For this review, take the finished solid that the model builds, in its own axes (mm). A direction names the side the tool comes from. Give positions to 0.01 mm unless a question says otherwise; leave off trailing zeros. Write each loop counter-clockwise with the first axis right and the second up, starting at its lowest first coordinate (ties: lowest second). Pieces come first, ordered by that corner, then holes. Notation, with made-up numbers: M -3.75,-36 L 35.25,-36 A33 cw 35.25,0 Z; hole C 72.5,80.25 d8. An arc over 180 degrees is marked long. Answer as a JSON object with one key per item and string values. Group by question number.
```python
from build123d import *

# Parameters (mm, degrees)
EXTRUDE_1_DEPTH     = 10
CUT_EXTRUDE_1_DEPTH = 3.6
SKETCH_3_R          = 4
CUT_EXTRUDE_2_DEPTH = 1.6


with BuildPart() as part:
    # Эскиз1 → Бобышка-Вытянуть1 (new body)
    with BuildSketch(Plane.XY):
        Polygon((2.5, 0), (-2.5, 0), (-5, 1.7), (-5, 3.7), (5, 3.7), (5, 1.7), align=None)
    extrude(amount=EXTRUDE_1_DEPTH)

    # Эскиз2 → Вырез-Вытянуть1 (cut)
    with BuildSketch(Plane(origin=(0, 3.7, 0), x_dir=(1, 0, 0), z_dir=(0, 1, 0))):
        Polygon((2.75, -6.58771324), (2.75, -3.41228676), (0, -1.824573519), (-2.75, -3.41228676), (-2.75, -6.58771324), (0, -8.175426481), align=None)
    extrude(amount=-CUT_EXTRUDE_1_DEPTH, mode=Mode.SUBTRACT)

    # Эскиз3 → Вырез-Вытянуть2 (cut)
    with BuildSketch(Plane(origin=(0, 3.7, 0), x_dir=(1, 0, 0), z_dir=(0, 1, 0))):
        with Locations(Location((0, -5, 0), (0, 0, 270))):
            Circle(SKETCH_3_R)
    extrude(amount=-CUT_EXTRUDE_2_DEPTH, mode=Mode.SUBTRACT)


solid = part.part
```
Item 1: Machinability: for faces 1 (the flat face through (-2.75, 1, 5)), 2 (the flat face through (-1, 2.1, 2)), 3 (the flat face through (-5, 3, 5)), which of the approach directions +Z, -Z, +X, -X, +Y, -Y give a long, thin tool a straight path to every point of the face, cutting with its end or side? Answer none if there is none.
Item 2: Consider section A-A (z = 5). Give the boundary of the cut face in (x, y).
Item 3: To check wall thickness, follow probe 1 along X at (y, z) = (3.25, 5); probe 2 along Y at (x, z) = (1.75, 2.5); probe 3 along X at (y, z) = (1.2, 5). State the ranges of each line that lie inside material, in increasing order.
Item 4: Consider section D-D (y = 1.2). Give the boundary of the cut face in (x, z).
Item 5: Draft analysis for pull direction X (two halves, no side actions). For faces 4 (the flat face through (0, 2, 10)), 5 (the flat face through (1.36, 1.11, 7.39)), 6 (the flat face through (5, 3, 5)), state which applies: released by +X, released by -X, zero draft, split by the parting line, or undercut.
Item 6: Consider section B-B (y = 1.95). Give the boundary of the cut face in (x, z), plus the area to 3 significant figures.
Item 7: Consider section C-C (x = 1). Give the boundary of the cut face in (y, z), plus the area to 3 significant figures.
Item 8: Insertion check: P1, Ø3, axis at x = 0, z = 5.5, coming from the +Y side. The pin has a flat end and moves straight along its axis. Give the tip position at first contact, or say it passes through.
Result set:
{
 "1": {"face 1": "+Y, -Y", "face 2": "+Y", "face 3": "+Z, -Z, -X, +Y, -Y"},
 "2": {"outline": "M -5,1.7 L -2.75,0.17 L -2.75,2.1 L -4,2.1 L -4,3.7 L -5,3.7 Z; M -2.65,0.1 L -2.5,0 L 2.5,0 L 2.65,0.1 Z; M 2.75,0.17 L 5,1.7 L 5,3.7 L 4,3.7 L 4,2.1 L 2.75,2.1 Z"},
 "3": {"probe 1": "x = -5 to -4, 4 to 5", "probe 2": "y = 0 to 2.1", "probe 3": "x = -4.26 to -2.75, 2.75 to 4.26"},
 "4": {"outline": "M -4.26,0 L 4.26,0 L 4.26,10 L -4.26,10 Z; hole M -2.75,3.41 L 0,1.82 L 2.75,3.41 L 2.75,6.59 L 0,8.18 L -2.75,6.59 Z"},
 "5": {"face 4": "zero draft", "face 5": "undercut", "face 6": "released by +X"},
 "6": {"outline": "M -5,0 L 5,0 L 5,10 L -5,10 Z; hole M -2.75,3.41 L 0,1.82 L 2.75,3.41 L 2.75,6.59 L 0,8.18 L -2.75,6.59 Z", "area": "73.8 mm^2"},
 "7": {"outline": "M 0,0 L 3.7,0 L 3.7,1.13 L 2.1,1.13 L 2.1,2.4 L 0.1,2.4 L 0.1,7.6 L 2.1,7.6 L 2.1,8.87 L 3.7,8.87 L 3.7,10 L 0,10 Z", "area": "14.2 mm^2"},
 "8": {"P1": "stops at y = 0.1"}
}
